from build123d import *

# Parameters (mm, degrees)
CYLINDER268_R          = 2
CYLINDER268_DEPTH      = 26
CYLINDER267_R          = 32.5
CYLINDER267_DEPTH      = 26
CUT248_PLACEMENT_ANGLE = 90


with BuildPart() as cylinder268:
    # Cylinder268 → Cylinder268 (new body)
    with BuildSketch(Plane.XY):
        Circle(CYLINDER268_R)
    extrude(amount=CYLINDER268_DEPTH)


with BuildPart() as cut248:
    # Cylinder267 → Cylinder267 (new body)
    with BuildSketch(Plane(origin=(3, 0, 0), x_dir=(1, 0, 0), z_dir=(0, 0, 1))):
        Circle(CYLINDER267_R)
    extrude(amount=CYLINDER267_DEPTH)

    # Cut248: cut Cylinder268
    add(cylinder268.part, mode=Mode.SUBTRACT)


with BuildPart() as cut248_1:
    # Cut248 placement: moved
    add(cut248.part.moved(Location((47, 54, 10))).rotate(Axis((47, 54, 10), (0, 1, 0)), CUT248_PLACEMENT_ANGLE))


solid = cut248_1.part
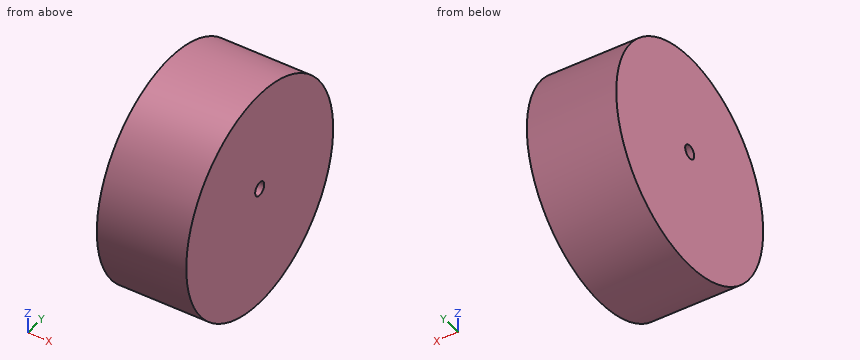
Geometry check sheet. Reference: the model listing, model coordinates, mm. Coordinates: 2 decimals unless noted, no trailing zeros. Loops run counter-clockwise (first coordinate to the right, second up) from the corner with the lowest first, then second, coordinate; pieces in that order, holes last. Notation, with made-up numbers: (88.5, -20.75) - (125.5, -20.75) arc R26 cw to (125.5, 18.25) - close; hole circle Ø3 at (-2.75, 14). An arc over 180 degrees is marked (long way). Use one line per item in the form item = value. Start each with the question number.
Item 1: Section check C-C, the plane x = 50. Enter the section's corners in (y, z), and give its area (3 significant figures).
Item 2: Thickness scan on probe 1 along Y at (x, z) = (67, 10); probe 2 along Y at (x, z) = (54.25, 29.5); probe 3 along Z at (x, y) = (61.25, 59.5). Record the ranges inside material, lowest first.
Item 3: Section check D-D, the plane z = -21. Enter the section's corners in (x, y).
Item 4: Gauge pin test, flat ends, axial feed: pin 1 (5 mm diameter, centred on x = 64, z = -14.5, fed in from +Y); pin 2 (8 mm diameter, centred on x = 61.5, y = 46, fed in from +Z); pin 3 (4 mm diameter, centred on x = 60.5, y = 65, fed in from -Z). Record the tip position at first contact, or that the pin passes through.
Item 5: Section check A-A, the plane y = 54. Enter the section's corners in (x, z), and give its area (3 significant figures).
Item 6: Section check B-B, the plane z = 10. Enter the section's corners in (x, y).
Computed:
q1.outline = circle Ø65 at (54, 7); hole circle Ø4 at (54, 10)
q1.area = 3,310 mm2
q2.probe_1 = 21.64 to 52, 56 to 86.36
q2.probe_2 = 30.55 to 77.45
q2.probe_3 = -25.03 to 39.03
q3.outline = (47, 37.5) - (73, 37.5) - (73, 70.5) - (47, 70.5) - close
q4.pin_1 = 80.37
q4.pin_2 = 39.25
q4.pin_3 = -24.23
q5.outline = (47, -25.5) - (73, -25.5) - (73, 8) - (47, 8) - close; (47, 12) - (73, 12) - (73, 39.5) - (47, 39.5) - close
q5.area = 1,590 mm2
q6.outline = (47, 21.64) - (73, 21.64) - (73, 52) - (47, 52) - close; (47, 56) - (73, 56) - (73, 86.36) - (47, 86.36) - close
